Work out the finished part from the listing and answer in its coordinate system (mm). A direction names the side the tool comes from. Round coordinates to 2 decimals unless told otherwise and drop trailing zeros. Order: outer loops, then holes, each group sorted by start corner. A loop starts at its lowest first (then second) coordinate and runs counter-clockwise, first axis right, second up. Notation, with made-up numbers: (83, 41.5) -> (133, 41.5) arc R22 cw to (133, 74.5) -> close; hole circle Ø5 at (72, -24). An arc over 180 degrees is marked (long way). Use a Markdown table: item, result. Add a question column.
Item 1: A cutting plane is placed at C-C, the plane z = 0. Determine the outline of the cut face in (x, y).
Item 2: A cutting plane is placed at A-A, the plane y = 8.75. Determine the outline of the cut face in (x, z).
Item 3: For a pull along Z with two mould halves and no side action, classify faces 1 (the flat face through (4, 0, -6.5)), 2 (the cylindrical face through (8.226, 1.072, 3.405)), 3 (the flat face through (4, 0, -10)), 4 (the flat face through (-10, 4, 5)) as +Z half, -Z half, draft (parallel to the pull), parting line (faces both ways), or undercut.
Item 4: Flat-ended cylindrical pins translate along their axes: P1, Ø5.5, axis at x = 2, y = 1.5, coming from the +Z side; P2, Ø6.5, axis at y = 0, z = 0, coming from the -X side; P3, Ø5.5, axis at y = -0.5, z = -2, coming from the -X side. Find the tip coordinate at first contact, or state that the pin passes through.
Item 5: A cutting plane is placed at B-B, the plane x = 8.75. Determine the outline of the cut face in (y, z).
Item 6: A tool of negligible diameter and unlimited length cuts with its end or side. For faces 5 (the flat face through (4, -6.5, 0)), 6 (the flat face through (6.5, 0, 4)), 7 (the cylindrical face through (-4.05, 3.72, 7.67)), from which of +Z, -Z, +X, -X, +Y, -Y can it reach the whole face along a straight path? Write none if from no direction.
Item 7: Find the intervals of material crossed by L1, parallel to Z at x = 0, y = -9.1; L2, parallel to X at y = 0, z = -5.6, in increasing order. Write a range as [from, to].
from build123d import *

# Parameters (mm, degrees)
SKETCH1_W           = 20
SKETCH1_H           = 20
BOSS_EXTRUDE1_DEPTH = 10
SKETCH2_R           = 3.57
CUT_EXTRUDE1_DEPTH  = 21
SKETCH3_R           = 5.5
CUT_EXTRUDE2_DEPTH  = 16.5
SKETCH4_R           = 3.57
CUT_EXTRUDE3_DEPTH  = 21
SKETCH5_R           = 5.5
CUT_EXTRUDE4_DEPTH  = 16.5
SKETCH6_R           = 3.57
CUT_EXTRUDE5_DEPTH  = 21
SKETCH7_R           = 5.5
CUT_EXTRUDE6_DEPTH  = 16.5


with BuildPart() as part:
    # Sketch1 → Boss-Extrude1 (new body, symmetric)
    with BuildSketch(Plane.XY):
        Rectangle(SKETCH1_W, SKETCH1_H)
    extrude(amount=BOSS_EXTRUDE1_DEPTH, both=True)

    # Sketch2 → Cut-Extrude1 (cut, through all)
    with BuildSketch(Plane.XY.offset(10)):
        Circle(SKETCH2_R)
    extrude(amount=-CUT_EXTRUDE1_DEPTH, mode=Mode.SUBTRACT)

    # Sketch3 → Cut-Extrude2 (cut)
    with BuildSketch(Plane.XY.offset(10)):
        Circle(SKETCH3_R)
    extrude(amount=-CUT_EXTRUDE2_DEPTH, mode=Mode.SUBTRACT)

    # Sketch4 → Cut-Extrude3 (cut, through all)
    with BuildSketch(Plane.ZY.offset(10)):
        Circle(SKETCH4_R)
    extrude(amount=-CUT_EXTRUDE3_DEPTH, mode=Mode.SUBTRACT)

    # Sketch5 → Cut-Extrude4 (cut)
    with BuildSketch(Plane.ZY.offset(10)):
        Circle(SKETCH5_R)
    extrude(amount=-CUT_EXTRUDE4_DEPTH, mode=Mode.SUBTRACT)

    # Sketch6 → Cut-Extrude5 (cut, through all)
    with BuildSketch(Plane(origin=(0, 10, 0), x_dir=(1, 0, 0), z_dir=(0, 1, 0))):
        Circle(SKETCH6_R)
    extrude(amount=-CUT_EXTRUDE5_DEPTH, mode=Mode.SUBTRACT)

    # Sketch7 → Cut-Extrude6 (cut)
    with BuildSketch(Plane(origin=(0, 10, 0), x_dir=(1, 0, 0), z_dir=(0, 1, 0))):
        Circle(SKETCH7_R)
    extrude(amount=-CUT_EXTRUDE6_DEPTH, mode=Mode.SUBTRACT)


solid = part.part
Reported:
| question | item | result |
|---|---|---|
| 1 | outline | (-10, -10) -> (-3.57, -10) -> (-3.57, -6.5) -> (-5.5, -6.5) -> (-5.5, -5.5) -> (-10, -5.5) -> close; (-10, 5.5) -> (-5.5, 5.5) -> (-5.5, 10) -> (-10, 10) -> close; (3.57, -10) -> (10, -10) -> (10, -3.57) -> (6.5, -3.57) -> (6.5, -5.5) -> (5.5, -5.5) -> (5.5, -6.5) -> (3.57, -6.5) -> close; (5.5, 5.5) -> (6.5, 5.5) -> (6.5, 3.57) -> (10, 3.57) -> (10, 10) -> (5.5, 10) -> close |
| 2 | outline | (-10, -10) -> (10, -10) -> (10, 10) -> (-10, 10) -> close; hole circle Ø11 at (0, 0) |
| 3 | face 1 | +Z half |
| 3 | face 2 | undercut |
| 3 | face 3 | -Z half |
| 3 | face 4 | draft |
| 4 | P1 | z = -6.5 |
| 4 | P2 | through |
| 4 | P3 | x = 6.5 |
| 5 | outline | (-10, -10) -> (10, -10) -> (10, 10) -> (-10, 10) -> close; hole circle Ø7.14 at (0, 0) |
| 6 | face 5 | +Y |
| 6 | face 6 | -X |
| 6 | face 7 | +Z |
| 7 | L1 | [-10, -3.57], [3.57, 10] |
| 7 | L2 | [-10, -5.5], [5.5, 10] |
